Check sheet for the modelled part. Datum: model origin and axes. Units: mm. Face numbers are marked on the shaded views. A direction names the side the tool comes from. Coordinates: 2 decimals unless noted, no trailing zeros. Write each loop counter-clockwise with the first axis right and the second up, starting at its lowest first coordinate (ties: lowest second). Pieces come first, ordered by that corner, then holes. Notation, with made-up numbers: (53, 47) -> (82, 47) arc R12 ccw to (82, 62) -> close; hole circle Ø3 at (70, 17.5). An arc over 180 degrees is marked (long way). Put each result on its own line as item: value.
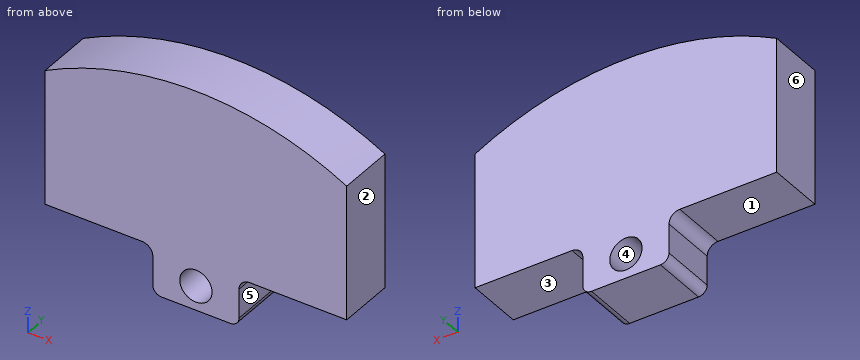
```python
from build123d import *

# Parameters (mm, degrees)
BOSS_EXTRUDE2_DEPTH = 13.335
SKETCH10_W          = 25.4
SKETCH10_H          = 11.43
CUT_EXTRUDE1_DEPTH  = 14.335
FILLET1_R           = 2.54
FILLET2_R           = 2.032
SKETCH11_R          = 3.81
CUT_EXTRUDE2_DEPTH  = 14.335


with BuildPart() as part:
    # Sketch6 → Boss-Extrude2 (new body)
    with BuildSketch(Plane(origin=(0, 0, 0), x_dir=(1, 0, 0), z_dir=(0, 1, 0))):
        with BuildLine():
            Line((0, 0), (71.12, 0))
            Line((71.12, 0), (71.12, -43.18))
            ThreePointArc((71.12, -43.18), (35.56, -52.012400668), (0, -43.18))
            Line((0, -43.18), (0, 0))
        make_face()
    extrude(amount=BOSS_EXTRUDE2_DEPTH)

    # Sketch10 → Cut-Extrude1 (cut, through all)
    with BuildSketch(Plane(origin=(0, 13.335, 0), x_dir=(1, 0, 0), z_dir=(0, 1, 0))):
        with Locations((58.42, -5.715)):
            Rectangle(SKETCH10_W, SKETCH10_H)
        with Locations((12.7, -5.715)):
            Rectangle(SKETCH10_W, SKETCH10_H)
    extrude(amount=-CUT_EXTRUDE1_DEPTH, mode=Mode.SUBTRACT)

    # Fillet1
    fillet1_edges = [part.edges().sort_by_distance(p)[0] for p in [
        (25.4, 6.6675, 11.43),
        (45.72, 6.6675, 11.43),
    ]]
    fillet(fillet1_edges, radius=FILLET1_R)

    # Fillet2
    fillet2_edges = [part.edges().sort_by_distance(p)[0] for p in [
        (25.4, 6.6675, 0),
        (45.72, 6.6675, 0),
    ]]
    fillet(fillet2_edges, radius=FILLET2_R)

    # Sketch11 → Cut-Extrude2 (cut, through all)
    with BuildSketch(Plane.XZ):
        with Locations((35.56, 5.718912503)):
            Circle(SKETCH11_R)
    extrude(amount=-CUT_EXTRUDE2_DEPTH, mode=Mode.SUBTRACT)


solid = part.part
```
Q1. Depth check by flat-ended pin: P1, Ø5.5, axis at y = 6, z = 5, coming from the +X side; P2, Ø6, axis at x = 55.5, y = 1.5, coming from the -Z side; P3, Ø2, axis at x = 55.5, y = 7, coming from the +Z side. Enter the tip coordinate at first touch or a pass-through.
Recorded:
P1: stops at x = 45.72
P2: stops at z = 11.43
P3: stops at z = 49.61
Q2. Mould release check, pull along X, two halves, no side actions. Record for the marked faces 4, 5 and 6: released by +X, released by -X, zero draft, split by the parting line, or undercut.
Recorded:
face 4: undercut
face 5: released by +X
face 6: released by -X
Q3. Material ranges on line 1 along Z through (x, y) = (35.56, 4.5); line 2 along X through (y, z) = (8, 7); line 3 along Z through (x, y) = (38, 5.5), recorded low to high.
Recorded:
line 1: z = 0 to 1.91, 9.53 to 52.01
line 2: x = 25.4 to 31.97, 39.15 to 45.72
line 3: z = 0 to 2.79, 8.65 to 51.97
Q4. Cross-section at A-A (x = 35.56). Record the cut outline in (y, z) (3 decimals), plus the area to 3 significant figures.
Recorded:
outline: (0, 0) -> (13.335, 0) -> (13.335, 1.909) -> (0, 1.909) -> close; (0, 9.529) -> (13.335, 9.529) -> (13.335, 52.012) -> (0, 52.012) -> close
area: 592 mm2
Q5. Cross-section at B-B (y = 7). Record the cut outline in (x, z).
Recorded:
outline: (0, 11.43) -> (22.86, 11.43) arc R2.54 cw to (25.4, 8.89) -> (25.4, 2.03) arc R2.03 ccw to (27.43, 0) -> (43.69, 0) arc R2.03 ccw to (45.72, 2.03) -> (45.72, 8.89) arc R2.54 cw to (48.26, 11.43) -> (71.12, 11.43) -> (71.12, 43.18) arc R76 ccw to (0, 43.18) -> close; hole circle Ø7.62 at (35.56, 5.72)
Q6. Cross-section at C-C (x = 50.5). Record the cut outline in (y, z) (3 decimals), plus the area to 3 significant figures.
Recorded:
outline: (0, 11.43) -> (13.335, 11.43) -> (13.335, 50.529) -> (0, 50.529) -> close
area: 521 mm2
Q7. Tool access check on the marked faces 1, 2 and 3. Record the directions out of +Z, -Z, +X, -X, +Y, -Y that give a thin tool (end or side, any length) a straight path to the whole face; none if there is none.
Recorded:
face 1: -Z, -X, +Y, -Y
face 2: +Z, -Z, +X, +Y, -Y
face 3: -Z, +X, +Y, -Y
